Check sheet for the modelled part. Datum: model origin and axes. Units: mm. A direction names the side the tool comes from. Give positions to 0.01 mm unless a question says otherwise; leave off trailing zeros. Loops run counter-clockwise (first coordinate to the right, second up) from the corner with the lowest first, then second, coordinate; pieces in that order, holes last. Notation, with made-up numbers: (44.25, 66.5) -> (94.25, 66.5) arc R20 ccw to (94.25, 105.5) -> close; hole circle Ø7 at (-7.75, 59). An arc over 180 degrees is marked (long way). Answer as CSV lines item,"result". Start each with the question number.
(1) Section check A-A on y = 7.75. Enter the section's corners in (x, z).
(2) Release check for a two-part mould opening along Z. For faces 1 (the face through (25, 8, -203.2)), 2 (the face through (25, 10, -4.648)), 3 (the face through (49.35, 14.17, -200.91)), 4 (the face through (25, 8, 0)) record: pulls with the +Z half, pulls with the -Z half, needs draft (parallel to the pull), parting line crosses it, or undercut.
(3) Access from +Z, -Z, +X, -X, +Y, -Y to the whole of each face (thin tool, end or side, straight path). Record for faces 5 (the face through (1.45, 14.17, -2.36)), 6 (the face through (25, 4.648, -103)).
(4) Section check B-B on x = 24.5. Enter the section's corners in (y, z).
(5) Section check C-C on z = -106. Enter the section's corners in (x, y), plus the area to 3 significant figures.
(6) Gauge pin test, flat end, axial feed: pin 1 Ø10 at (x, z) = (43, -71) entering from +Y. Record the tip position at first contact, or that the pin passes through.
(7) Material ranges on line 1 (Z direction, x = 27, y = 6.75); line 2 (Y direction, x = 8.5, z = -155.5), recorded low to high. Write a range as from..to.
from build123d import *

# Parameters (mm, degrees)
SKETCH1_W           = 50.8
SKETCH1_H           = 203.2
BOSS_EXTRUDE1_DEPTH = 4.6482
SKETCH2_W           = 50.8
SKETCH2_H           = 4.6482
BOSS_EXTRUDE2_DEPTH = 11.049
FILLET1_R           = 5.08


with BuildPart() as part:
    # Sketch1 → Boss-Extrude1 (new body)
    with BuildSketch(Plane(origin=(0, 0, 0), x_dir=(1, 0, 0), z_dir=(0, 1, 0))):
        with Locations((25.4, 101.6)):
            Rectangle(SKETCH1_W, SKETCH1_H)
    extrude(amount=BOSS_EXTRUDE1_DEPTH)

    # Sketch2 → Boss-Extrude2 (add)
    with BuildSketch(Plane(origin=(0, 4.6482, 0), x_dir=(1, 0, 0), z_dir=(0, 1, 0))):
        with Locations((25.4, 2.3241)):
            Rectangle(SKETCH2_W, SKETCH2_H)
        with Locations((25.4, 200.8759)):
            Rectangle(SKETCH2_W, SKETCH2_H)
    extrude(amount=BOSS_EXTRUDE2_DEPTH)

    # Fillet1
    fillet1_edges = [part.edges().sort_by_distance(p)[0] for p in [
        (0, 15.6972, -2.3241),
        (50.8, 15.6972, -2.3241),
        (0, 15.6972, -200.8759),
        (50.8, 15.6972, -200.8759),
    ]]
    fillet(fillet1_edges, radius=FILLET1_R)


solid = part.part
Working result:
1,outline,"(0, -203.2) -> (50.8, -203.2) -> (50.8, -198.55) -> (0, -198.55) -> close; (0, -4.65) -> (50.8, -4.65) -> (50.8, 0) -> (0, 0) -> close"
2,face 1,"pulls with the -Z half"
2,face 2,"undercut"
2,face 3,"needs draft"
2,face 4,"pulls with the +Z half"
3,face 5,"+Z, -Z, -X, +Y"
3,face 6,"+X, -X, +Y"
4,outline,"(0, -203.2) -> (15.7, -203.2) -> (15.7, -198.55) -> (4.65, -198.55) -> (4.65, -4.65) -> (15.7, -4.65) -> (15.7, 0) -> (0, 0) -> close"
5,outline,"(0, 0) -> (50.8, 0) -> (50.8, 4.65) -> (0, 4.65) -> close"
5,area,"236 mm^2"
6,pin 1,"stops at y = 4.65"
7,line 1,"z = -203.2..-198.55, -4.65..0"
7,line 2,"y = 0..4.65"
